CAD build for the part. Positions are in the model's coordinates, mm. A direction names the side the tool comes from. Coordinates: 2 decimals unless noted, no trailing zeros. Order: outer loops, then holes, each group sorted by start corner. A loop starts at its lowest first (then second) coordinate and runs counter-clockwise, first axis right, second up. Notation, with made-up numbers: M 62.25,59 L 97.25,59 A16 cw 97.25,86 Z; hole C 47.5,78 d8. An arc over 180 degrees is marked long. One line per item, written item: value.
Autodesk Inventor part; units mm, degrees
ref_plane "YZ Plane" through (0, 0, 0) normal (1, 0, 0) x (0, 1, 0)
ref_plane "XZ Plane" through (0, 0, 0) normal (0, 1, 0) x (-1, 0, 0)
ref_plane "XY Plane" through (0, 0, 0) normal (0, 0, 1) x (1, 0, 0)
sketch "Sketch1" plane through (0, 0, 0) normal (0, 0, 1) x (1, 0, 0)
  line L0 (0, 0) -> (0, -10.95)
  line L1 (0, -10.95) -> (6.925, -10.95)
  line L2 (6.925, -10.95) -> (6.925, -7.8)
  line L3 (6.925, -7.8) -> (5, -7.8)
  line L4 (5, -7.8) -> (5, -3)
  line L5 (5, -3) -> (9, -3)
  line L6 (9, -3) -> (9, 0)
  line L7 (9, 0) -> (0, 0)
  dimension "d0" = 6.925
  dimension "d1" = 5
  dimension "d2" = 9
  dimension "d3" = 3.15
  dimension "d4" = 4.8
  dimension "d5" = 3
revolve "Revolution1" add sketch "Sketch1" angle 360 about axis through (0, 0, 0) along (0, -1, 0)
sketch "Sketch2" plane through (0, 0, 0) normal (0, 1, 0) x (1, 0, 0)
  circle A0 centre (0, 0) radius 9
  line L0 (0, 12.6) -> (0, -12.6)
  line L1 (7.5, 4.9749) -> (7.5, -4.9749)
  line L2 (-7.5, 4.9749) -> (-7.5, -4.9749)
  dimension "d7" = 15
  dimension "d8" = 7.5
extrude "Extrusion1" cut sketch "Sketch2" against normal up to surface (3 mm away) contours A0 L1 | L2 A0
sketch "Sketch3" plane through (0, -3, 0) normal (0, -1, 0) x (1, 0, 0)
  arc A0 (-7.5, -4.9749) -> (7.5, -4.9749) centre (0, 0) ccw
  line L0 (7.5, -4.9749) -> (7.5, 4.9749)
  circle A1 centre (0, 0) radius 5
  line L1 (-4, -3) -> (-4, 3)
  line L2 (4, -3) -> (4, 3)
  dimension "d11" = 8
  dimension "d12" = 4
extrude "Extrusion2" cut sketch "Sketch3" along normal up to surface (4.8 mm away) contours A1 L2 | L1 A1
fillet "Fillet1" radius 1 4 edges at (4, -5.4, 3) (4, -5.4, -3) (-4, -5.4, 3) (-4, -5.4, -3)
fillet "Fillet2" radius 1.5 4 edges at (7.5, -1.5, 4.9749) (7.5, -1.5, -4.9749) (-7.5, -1.5, 4.9749) (-7.5, -1.5, -4.9749)
equation "\"d8\" = 0.5 * d7"
equation "\"d12\" = 0.5 * d11"
properties part number "318-06" material "Steel"
Q1. Slice it at B-B (y = -4.5). List the corners of the cut face in (x, z), plus the area to 3 significant figures.
Recorded:
outline: M -4,-2.65 A1 ccw -3.75,-3.31 A5 ccw 3.75,-3.31 A1 ccw 4,-2.65 L 4,2.65 A1 ccw 3.75,3.31 A5 ccw -3.75,3.31 A1 ccw -4,2.65 Z
area: 70.3 mm^2
Q2. Slice it at D-D (x = -4.5). List the corners of the cut face in (y, z).
Recorded:
outline: M -10.95,-5.26 L -7.8,-5.26 L -7.8,5.26 L -10.95,5.26 Z; M -3,-7.79 L 0,-7.79 L 0,7.79 L -3,7.79 Z
Q3. Slice it at C-C (z = 0). List the corners of the cut face in (x, y) (3 decimals).
Recorded:
outline: M -7.5,-3 L -4,-3 L -4,-7.8 L -6.925,-7.8 L -6.925,-10.95 L 6.925,-10.95 L 6.925,-7.8 L 4,-7.8 L 4,-3 L 7.5,-3 L 7.5,0 L -7.5,0 Z
Q4. Mould opens along Y. For faces 1 (the face through (-7.42, -1.52, 4.98)), 2 (the face through (-4, -5, 0)), 3 (the face through (0, 0, 0)) say: released by +Y, released by -Y, zero draft, split by the parting line, or undercut.
Recorded:
face 1: zero draft
face 2: undercut
face 3: released by +Y
Q5. Drill centre lines: line 1 along Y through (x, z) = (0, -5.75); line 2 along Y through (x, z) = (-3.5, 6.25); line 3 along X through (y, z) = (-4.5, -1.25). Where is each one in solid material? Low to high.
Recorded:
line 1: y = -10.95 to -7.8, -3 to 0
line 2: y = -3 to 0
line 3: x = -4 to 4
Q6. Slice it at A-A (x = 0). List the corners of the cut face in (y, z) (3 decimals).
Recorded:
outline: M -10.95,-6.925 L -7.8,-6.925 L -7.8,-5 L -3,-5 L -3,-9 L 0,-9 L 0,9 L -3,9 L -3,5 L -7.8,5 L -7.8,6.925 L -10.95,6.925 Z
Q7. Pin check, flat tips, straight feed: pin 1 Ø5 at (y, z) = (-6.5, 4.5) entering from +X; pin 2 Ø2.5 at (y, z) = (-6, -1) entering from +X; pin 3 Ø1.5 at (y, z) = (-3, 6.5) entering from +X; pin 4 Ø8 at (x, z) = (4, -6.5) entering from -Y. Stop position of each tip, or through.
Recorded:
pin 1: stops at x = 6.51
pin 2: stops at x = 4
pin 3: stops at x = 6.92
pin 4: stops at y = -10.95
Q8. Which spindle directions (+Z, -Z, +X, -X, +Y, -Y) get a long thin tool onto all of the face, cutting with end or side? Do faces 4 (the face through (5, -7.8, 0)), 5 (the face through (0, -5, -5)), 6 (the face through (4, -5, 0)), 7 (the face through (0, -5, 5)), 8 (the face through (6.6, -9.4, -2.1)). Say none if no direction does.
Recorded:
face 4: none
face 5: -Z
face 6: +Z, -Z, +X
face 7: +Z
face 8: -Y
